Work out the finished part from the listing and answer in its coordinate system (mm). A direction names the side the tool comes from. Round coordinates to 2 decimals unless told otherwise and drop trailing zeros. Order: outer loops, then holes, each group sorted by start corner. A loop starts at its lowest first (then second) coordinate and runs counter-clockwise, first axis right, second up.
from build123d import *

# Parameters (mm, degrees)
BOSS_EXTRUDE1_DEPTH = 9
SKETCH2_W           = 206.758876678
SKETCH2_H           = 6
CUT_EXTRUDE1_DEPTH  = 7


with BuildPart() as part:
    # Sketch1 → Boss-Extrude1 (new, symmetric)
    with BuildSketch(Plane.XY):
        Polygon((-28, 0), (28, 0), (28, 13), (18, 23), (-18, 23), (-28, 5.679491924), align=None)
    extrude(amount=BOSS_EXTRUDE1_DEPTH, both=True)

    # Sketch2 → Cut-Extrude1 (cut)
    with BuildSketch(Plane(origin=(0, 23, 0), x_dir=(1, 0, 0), z_dir=(0, 1, 0))):
        Rectangle(SKETCH2_W, SKETCH2_H)
    extrude(amount=-CUT_EXTRUDE1_DEPTH, mode=Mode.SUBTRACT)


solid = part.part
Item 1: Find section C-C (y = 16.75). Write down the section's boundary in (x, z), plus the area to 3 significant figures.
Item 2: Find the intervals of material crossed by line 1 along Z through (x, y) = (2, 17.75); line 2 along Y through (x, z) = (3, -1); line 3 along Y through (x, z) = (-20, -4.75), in increasing order.
Item 3: For a pull along Z with two mould halves and no side action, classify faces 1 (the face through (1, 16, 0)), 2 (the face through (0, 12, -9)), 3 (the face through (0, 12, 9)), 4 (the face through (-28, 3, 0)) as released by +Z, released by -Z, zero draft, split by the parting line, or undercut.
Item 4: Find section D-D (z = -5). Write down the section's boundary in (x, y).
Item 5: Find section A-A (z = 1.75). Write down the section's boundary in (x, y), plus the area to 3 significant figures.
Item 6: Given pin 1 (6 mm diameter, centred on y = 14.5, z = 7, fed in from -X); pin 2 (4 mm diameter, centred on y = 13, z = -4, fed in from -X); pin 3 (4 mm diameter, centred on x = 21.5, z = 5.5, fed in from +Y), each flat-ended and moving along its own axis, determine where each tip first touches the part or whether it passes through.
Item 7: Find section B-B (x = -8.5). Write down the section's boundary in (y, z), plus the area to 3 significant figures.
Item 8: A tool of negligible diameter and unlimited length cuts with its end or side. For faces 5 (the face through (1, 20, 3)), 6 (the face through (-22.93, 14.46, 0.13)), from which of +Z, -Z, +X, -X, +Y, -Y can it reach the whole face along a straight path? Write none if from no direction.
Model answer:
1. outline: (-21.61, -9) - (24.25, -9) - (24.25, -3) - (-21.61, -3) - close; (-21.61, 3) - (24.25, 3) - (24.25, 9) - (-21.61, 9) - close
1. area: 550 mm2
2. line 1: z = -9 to -3, 3 to 9
2. line 2: y = 0 to 16
2. line 3: y = 0 to 19.54
3. face 1: undercut
3. face 2: released by -Z
3. face 3: released by +Z
3. face 4: zero draft
4. outline: (-28, 0) - (28, 0) - (28, 13) - (18, 23) - (-18, 23) - (-28, 5.68) - close
5. outline: (-28, 0) - (28, 0) - (28, 13) - (25, 16) - (-22.04, 16) - (-28, 5.68) - close
5. area: 861 mm2
6. pin 1: stops at x = -24.64
6. pin 2: stops at x = -24.93
6. pin 3: stops at y = 21.5
7. outline: (0, -9) - (23, -9) - (23, -3) - (16, -3) - (16, 3) - (23, 3) - (23, 9) - (0, 9) - close
7. area: 372 mm2
8. face 5: +X, -X, +Y
8. face 6: +Z, -Z, -X, +Y
